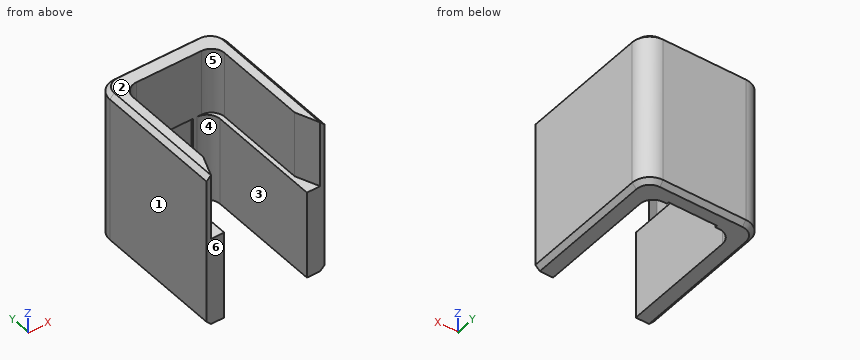
Autodesk Fusion 360 part; units mm, degrees
sketch "Sketch1" plane through (0, 0, 0) normal (0, 0, 1) x (1, 0, 0)
  line L0 (-9.35, 0) -> (-9.35, 29)
  line L1 (-10.35, 29) -> (0, 29)
  line L2 (0, 33) -> (-13.35, 33)
  line L3 (-13.35, 33) -> (-13.35, 0)
  line L4 (-13.35, 0) -> (-9.35, 0)
  line L5 (-10.35, 0) -> (-10.35, 29)
  line L6 (0, 2.5) -> (0, 20)
  line L7 (13.35, 0) -> (9.35, 0)
  line L8 (0, 33) -> (13.35, 33)
  line L9 (13.35, 33) -> (13.35, 0)
  line L10 (10.35, 0) -> (10.35, 29)
  line L11 (10.35, 29) -> (0, 29)
  line L12 (9.35, 0) -> (9.35, 29)
  line L13 (5.5, 29.5) -> (-5.5, 29.5)
  line L14 (-5.5, 29.5) -> (-5.5, 28.5)
  line L15 (-5.5, 28.5) -> (5.5, 28.5)
  line L16 (5.5, 28.5) -> (5.5, 29.5)
  line L17 (5.5, 29.5) -> (-5.5, 28.5) construction
  line L18 (-5.5, 29.5) -> (5.5, 28.5) construction
  point P0 (0, 29)
  dimension "d1" = 9.35
  dimension "d3" = 4
  dimension "d4" = 4
  dimension "d5" = 29
  dimension "d18" = 1
  dimension "d19" = 11
  dimension "d20" = 1
extrude "Extrude1" add sketch "Sketch1" against normal blind 20 contours L0 L1 L4 L5 | L1 L2 L3 L4 L5 L7 L8 L9 L10 L11 L13 L14 L16 | L7 L10 L11 L12
extrude "Extrude2" add sketch "Sketch1" along normal blind 15 contours L1 L2 L3 L4 L5 L7 L8 L9 L10 L11 L13 L14 L16 | L1 L11 L13 L14 L16
chamfer "Chamfer1" distance 2 distance2 5 1 edges at (-10.35, 0, 7.5) measured on face at (-11.0167, 0, -13.3333)
chamfer "Chamfer1" distance 5 distance2 2 1 edges at (10.35, 0, 7.5) measured on face at (10.35, 9.6667, 5)
fillet "Fillet1" radius 4 2 edges at (-13.35, 33, -2.5) (13.35, 33, -2.5)
fillet "Fillet2" radius 3 4 edges at (-9.35, 29, -10) (-10.35, 29, 7.5) (9.35, 29, -10) (10.35, 29, 7.5)
chamfer "Chamfer3" distance 1 angle 45 10 edges at (-13.35, 14.5, -20) (-12.1784, 31.8284, -20) (0, 33, -20) (12.1784, 31.8284, -20) (13.35, 14.5, -20) (-13.35, 14.5, 15) (13.35, 14.5, 15) (12.1784, 31.8284, 15) (0, 33, 15) (-12.1784, 31.8284, 15)
equation "d1 = ( 18.7 / 2 ) * 1 mm"
Part model, mm, in its own coordinate system. Face numbers are marked on the shaded views. A direction names the side the tool comes from. Give positions to 0.01 mm unless a question says otherwise; leave off trailing zeros. Loops run counter-clockwise (first coordinate to the right, second up) from the corner with the lowest first, then second, coordinate; pieces in that order, holes last. Notation, with made-up numbers: M -10,24 L 0,24 A33 ccw 0,55 Z; hole C 44.5,61.25 d1. An arc over 180 degrees is marked long. Return JSON: item names as keys, results as strings.
1) Saw through at B-B, the plane z = 4.5. List the corners of the cut face in (x, y), then the cut area to 3 significant figures.
Calculated:
{"outline": "M -13.35,0 L -12.35,0 L -10.35,5 L -10.35,26 A3 cw -7.35,29 L 7.35,29 A3 cw 10.35,26 L 10.35,5 L 12.35,0 L 13.35,0 L 13.35,29 A4 ccw 9.35,33 L -9.35,33 A4 ccw -13.35,29 Z", "area": "268 mm2"}
2) 3-axis set-ups, long thin cutter, end or side, ignore diameter. For the marked faces 4, 5 and 6: which of +Z, -Z, +X, -X, +Y, -Y reach the whole face in a straight line?
Calculated:
{"face 4": "+Z, -Z, -Y", "face 5": "+Z, -Y", "face 6": "+Z, -Z, +X, -X, -Y"}
3) Saw through at D-D, the plane y = 26.5. List the corners of the cut face in (x, z), then the cut area to 3 significant figures.
Calculated:
{"outline": "M -13.35,-19 L -12.35,-20 L -9.31,-20 L -9.31,0 L -10.31,0 L -10.31,15 L -12.35,15 L -13.35,14 Z; M 9.31,-20 L 12.35,-20 L 13.35,-19 L 13.35,14 L 12.35,15 L 10.31,15 L 10.31,0 L 9.31,0 Z", "area": "251 mm2"}
4) Pull direction X, two halves, no side cores. Call the marked faces 1, 2 and 3: released by +X, released by -X, zero draft, split by the parting line, or undercut.
Calculated:
{"face 1": "released by -X", "face 2": "zero draft", "face 3": "undercut"}
5) Saw through at C-C, the plane x = -3.75. List the corners of the cut face in (y, z), then the cut area to 3 significant figures.
Calculated:
{"outline": "M 29,0 L 29.5,0 L 29.5,-20 L 32,-20 L 33,-19 L 33,14 L 32,15 L 29,15 Z", "area": "129 mm2"}
6) Drill centre lines: line 1 (X direction, y = 19, z = 6.5); line 2 (X direction, y = 21, z = -5); line 3 (Y direction, x = -1.75, z = 4.5). Where is each one in solid material? Low to high.
Calculated:
{"line 1": "x = -13.35 to -10.35, 10.35 to 13.35", "line 2": "x = -13.35 to -9.35, 9.35 to 13.35", "line 3": "y = 29 to 33"}
7) Saw through at A-A, the plane y = 6. List the corners of the cut face in (x, z).
Calculated:
{"outline": "M -13.35,-19 L -12.35,-20 L -9.35,-20 L -9.35,0 L -10.35,0 L -10.35,15 L -12.35,15 L -13.35,14 Z; M 9.35,-20 L 12.35,-20 L 13.35,-19 L 13.35,14 L 12.35,15 L 10.35,15 L 10.35,0 L 9.35,0 Z"}
8) Flat gauge pins, fed straight in: pin 1 Ø3.5 at (x, z) = (0, -7) entering from -Y; pin 2 Ø8 at (x, y) = (-5.5, 28) entering from -Z. Where does each tip first touch, or does it go through?
Calculated:
{"pin 1": "stops at y = 29.5", "pin 2": "stops at z = -20"}
